from build123d import *

# Parameters (mm, degrees)
F0_W      = 120
F0_H      = 20
F1_DEPTH  = 3
F2_R      = 8
F3_DEPTH  = 2
F4_R      = 4.95
F4_R_2    = 4.15
F5_DEPTH  = 2.5
F5_FACE_R = 4.15
F6_DEPTH  = 0.4


with BuildPart() as f1:
    # F0 (on Top) → F1 (new body)
    with BuildSketch(Plane.XY):
        Rectangle(F0_W, F0_H)
    extrude(amount=F1_DEPTH)

    # F2 (on face) → F3 (cut)
    with BuildSketch(Plane.XY.offset(3)):
        with Locations((-40, 0)):
            Circle(F2_R)
    extrude(amount=-F3_DEPTH, mode=Mode.SUBTRACT)

    # F4 (on face) → F5 (join)
    with BuildSketch(Plane.XY.offset(1)):
        with Locations((-40, 0)):
            Circle(F4_R)
        with Locations((-40, 0)):
            Circle(F4_R_2, mode=Mode.SUBTRACT)
    extrude(amount=F5_DEPTH)

    # F5_face (on face) → F6 (join)
    with BuildSketch(Plane(origin=(-40, 0, 1), x_dir=(1, 0, 0), z_dir=(0, 0, 1))):
        Circle(F5_FACE_R)
    extrude(amount=F6_DEPTH)


solid = f1.part
The listing builds one solid part. Answer for the finished solid, in the listing's coordinates (mm). A direction names the side the tool comes from. Coordinates: 2 decimals unless noted, no trailing zeros. Loops run counter-clockwise (first coordinate to the right, second up) from the corner with the lowest first, then second, coordinate; pieces in that order, holes last. Notation, with made-up numbers: M 47,84 L 73,84 A8 cw 73,93 Z; hole C 18.25,19.5 d10. An arc over 180 degrees is marked long. Answer in a Markdown table with one row per item.
1) Given pin 1 (4 mm diameter, centred on x = 1, y = 6, fed in from -Z); pin 2 (6 mm diameter, centred on x = -19, y = -6.5, fed in from +Z), each flat-ended and moving along its own axis, determine where each tip first touches the part or whether it passes through.
Answers below:
| item | result |
|---|---|
| pin 1 | z = 0 |
| pin 2 | z = 3 |
2) Find section A-A (z = 2.4). Determine the outline of the cut face in (x, y), then the cut area to 3 significant figures.
Answers below:
| item | result |
|---|---|
| outline | M -60,-10 L 60,-10 L 60,10 L -60,10 Z; C -40,0 d9.9; hole C -40,0 d16; hole C -40,0 d8.3 |
| area | 2,220 mm^2 |
3) Determine the mould class of faces 1 (the cylindrical face through (-35.43, -1.9, 2.23)), 2 (the flat face through (-1, 0, 3)), 3 (the flat face through (-1, 10, 1)) for opening direction Y: released by +Y, released by -Y, zero draft, split by the parting line, or undercut.
Answers below:
| item | result |
|---|---|
| face 1 | undercut |
| face 2 | zero draft |
| face 3 | released by +Y |
4) Find the intervals of material crossed by probe 1 along Y at (x, z) = (-40, 1.8); probe 2 along Y at (x, z) = (-42, 2.55); probe 3 along X at (y, z) = (-2.75, 1.15), in increasing order.
Answers below:
| item | result |
|---|---|
| probe 1 | -10 to -8, -4.95 to -4.15, 4.15 to 4.95, 8 to 10 |
| probe 2 | -10 to -7.75, -4.53 to -3.64, 3.64 to 4.53, 7.75 to 10 |
| probe 3 | -60 to -47.51, -44.12 to -35.88, -32.49 to 60 |
5) Find section C-C (y = 0). Determine the outline of the cut face in (x, z), then the cut area to 3 significant figures.
Answers below:
| item | result |
|---|---|
| outline | M -60,0 L 60,0 L 60,3 L -32,3 L -32,1 L -35.05,1 L -35.05,3.5 L -35.85,3.5 L -35.85,1.4 L -44.15,1.4 L -44.15,3.5 L -44.95,3.5 L -44.95,1 L -48,1 L -48,3 L -60,3 Z |
| area | 335 mm^2 |
6) Which of the six approach directions +Z, -Z, +X, -X, +Y, -Y give full straight-line access (tool end or side, diameter ignored) to faces 4 (the cylindrical face through (-36.042, 1.247, 2.435)), 5 (the flat face through (-1, 0, 0))?
Answers below:
| item | result |
|---|---|
| face 4 | +Z |
| face 5 | -Z, +X, -X, +Y, -Y |
7) Find section B-B (x = -40). Determine the outline of the cut face in (y, z), then the cut area to 3 significant figures.
Answers below:
| item | result |
|---|---|
| outline | M -10,0 L 10,0 L 10,3 L 8,3 L 8,1 L 4.95,1 L 4.95,3.5 L 4.15,3.5 L 4.15,1.4 L -4.15,1.4 L -4.15,3.5 L -4.95,3.5 L -4.95,1 L -8,1 L -8,3 L -10,3 Z |
| area | 35.3 mm^2 |
8) Find section D-D (x = -21). Determine the outline of the cut face in (y, z).
Answers below:
| item | result |
|---|---|
| outline | M -10,0 L 10,0 L 10,3 L -10,3 Z |
